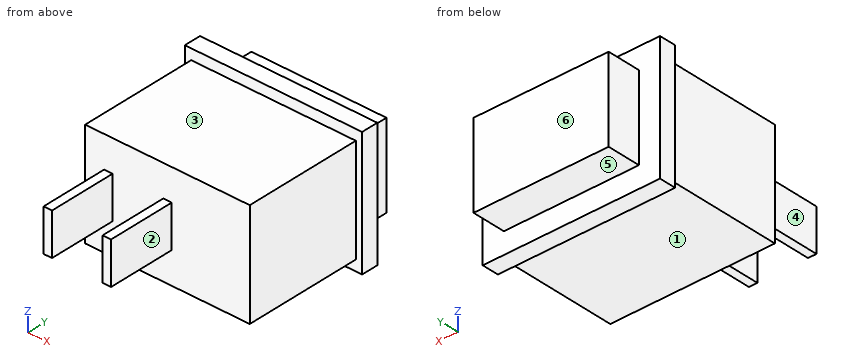
```python
from build123d import *

# Parameters (mm, degrees)
SKETCH_1_W      = 21
SKETCH_1_H      = 15
EXTRUDE_1_DEPTH = 2
SKETCH_2_W      = 16
SKETCH_2_H      = 10
EXTRUDE_2_DEPTH = 4
SKETCH_3_W      = 19.5
SKETCH_3_H      = 12.5
EXTRUDE_3_DEPTH = 14
SKETCH_4_W      = 1
SKETCH_4_H      = 5
EXTRUDE_4_DEPTH = 8


with BuildPart() as part:
    # Эскиз1 → Бобышка-Вытянуть1 (new body)
    with BuildSketch(Plane(origin=(0, 0, 0), x_dir=(1, 0, 0), z_dir=(0, 1, 0))):
        Rectangle(SKETCH_1_W, SKETCH_1_H)
    extrude(amount=EXTRUDE_1_DEPTH)

    # Эскиз2 → Бобышка-Вытянуть2 (add)
    with BuildSketch(Plane(origin=(0, 2, 0), x_dir=(1, 0, 0), z_dir=(0, 1, 0))):
        Rectangle(SKETCH_2_W, SKETCH_2_H)
    extrude(amount=EXTRUDE_2_DEPTH)

    # Эскиз3 → Бобышка-Вытянуть3 (add)
    with BuildSketch(Plane.XZ):
        Rectangle(SKETCH_3_W, SKETCH_3_H)
    extrude(amount=EXTRUDE_3_DEPTH)

    # Эскиз4 → Бобышка-Вытянуть4 (add)
    with BuildSketch(Plane.XZ.offset(14)):
        with Locations((-7, 0)):
            Rectangle(SKETCH_4_W, SKETCH_4_H)
        Rectangle(SKETCH_4_W, SKETCH_4_H)
    extrude(amount=EXTRUDE_4_DEPTH)


solid = part.part
```
Model file for the job. Use its own axes, mm. Face numbers are marked on the shaded views. A direction names the side the tool comes from. Give positions to 0.01 mm unless a question says otherwise; leave off trailing zeros. Loops run counter-clockwise (first coordinate to the right, second up) from the corner with the lowest first, then second, coordinate; pieces in that order, holes last. Notation, with made-up numbers: M 48,-0.5 L 106,-0.5 A26 ccw 106,29.5 Z; hole C -27,25.5 d11. An arc over 180 degrees is marked long. Use one line per item in the form item = value.
Item 1: Slice it at A-A on y = -15. List the corners of the cut face in (x, z).
Filled in:
outline = M -7.5,-2.5 L -6.5,-2.5 L -6.5,2.5 L -7.5,2.5 Z; M -0.5,-2.5 L 0.5,-2.5 L 0.5,2.5 L -0.5,2.5 Z
Item 2: Slice it at C-C on z = 3.5. List the corners of the cut face in (x, y).
Filled in:
outline = M -10.5,0 L -9.75,0 L -9.75,-14 L 9.75,-14 L 9.75,0 L 10.5,0 L 10.5,2 L 8,2 L 8,6 L -8,6 L -8,2 L -10.5,2 Z
Item 3: Slice it at D-D on y = 3. List the corners of the cut face in (x, z).
Filled in:
outline = M -8,-5 L 8,-5 L 8,5 L -8,5 Z
Item 4: Two-plate mould, pull along Y, no slides. Class the marked faces 5 and 6: released by +Y, released by -Y, zero draft, split by the parting line, or undercut.
Filled in:
face_5 = zero draft
face_6 = released by +Y
Item 5: Flat gauge pins, fed straight in: pin 1 Ø1 at (y, z) = (-15, 0) entering from +X; pin 2 Ø2.5 at (y, z) = (-17.5, -0.5) entering from -X; pin 3 Ø1.5 at (y, z) = (-7.5, 4) entering from -X; pin 4 Ø3 at (y, z) = (3, 2) entering from +X. Where does each tip first touch, or does it go through?
Filled in:
pin_1 = 0.5
pin_2 = -7.5
pin_3 = -9.75
pin_4 = 10.5
Item 6: Which spindle directions (+Z, -Z, +X, -X, +Y, -Y) get a long thin tool onto all of the face, cutting with end or side? Do the marked faces 1, 2, 3 and 4. Say none if no direction does.
Filled in:
face_1 = -Z, +X, -X, -Y
face_2 = +Z, -Z, +X, -Y
face_3 = +Z, +X, -X, -Y
face_4 = +Z, -Z, -X, -Y
Item 7: Drill centre lines: L1, parallel to X at y = -16, z = 1.5; L2, parallel to X at y = -8.5, z = -3.75; L3, parallel to Y at x = 2, z = -4.25. Where is each one in solid material? Low to high.
Filled in:
L1 = -7.5 to -6.5, -0.5 to 0.5
L2 = -9.75 to 9.75
L3 = -14 to 6
Item 8: Slice it at B-B on x = -6. List the corners of the cut face in (y, z).
Filled in:
outline = M -14,-6.25 L 0,-6.25 L 0,-7.5 L 2,-7.5 L 2,-5 L 6,-5 L 6,5 L 2,5 L 2,7.5 L 0,7.5 L 0,6.25 L -14,6.25 Z
